```python
from build123d import *

# Parameters (mm, degrees)
CYLINDER004_R               = 7
CYLINDER004_DEPTH           = 15
CYLINDER005_R               = 7
CYLINDER005_DEPTH           = 15
BOX006_W                    = 50
BOX006_H                    = 10
BOX006_DEPTH                = 4
CYLINDER007_R               = 4.5
CYLINDER007_DEPTH           = 4
CYLINDER007_PLACEMENT_ANGLE = 15
CYLINDER006_R               = 7
CYLINDER006_DEPTH           = 4
CYLINDER006_PLACEMENT_ANGLE = 15
BOX005_W                    = 10
BOX005_H                    = 10
BOX005_DEPTH                = 10
CYLINDER002_R               = 5
CYLINDER002_DEPTH           = 45
CYLINDER002_PLACEMENT_ANGLE = 60
BOX003_W                    = 10
BOX003_H                    = 40
BOX003_DEPTH                = 5
BOX003_PLACEMENT_ANGLE      = 30
CYLINDER003_R               = 6
CYLINDER003_DEPTH           = 20
CYLINDER003_PLACEMENT_ANGLE = 25
CYLINDER_R                  = 5
CYLINDER_DEPTH              = 50
BOX001_W                    = 50
BOX001_H                    = 40
BOX001_DEPTH                = 17
BOX001_PLACEMENT_ANGLE      = 30
BOX_W                       = 50
BOX_H                       = 40
BOX_DEPTH                   = 20
BOX004_W                    = 10
BOX004_H                    = 10
BOX004_DEPTH                = 10
CYLINDER001_R               = 5
CYLINDER001_DEPTH           = 45
CYLINDER001_PLACEMENT_ANGLE = 60
BOX002_W                    = 10
BOX002_H                    = 40
BOX002_DEPTH                = 5
BOX002_PLACEMENT_ANGLE      = 30


with BuildPart() as cylinder004:
    # Cylinder004 → Cylinder004 (new body)
    with BuildSketch(Plane(origin=(0, 36, 17), x_dir=(0, 0, -1), z_dir=(1, 0, 0))):
        Circle(CYLINDER004_R)
    extrude(amount=CYLINDER004_DEPTH)


with BuildPart() as cylinder005:
    # Cylinder005 → Cylinder005 (new body)
    with BuildSketch(Plane(origin=(35, 36, 17), x_dir=(0, 0, -1), z_dir=(1, 0, 0))):
        Circle(CYLINDER005_R)
    extrude(amount=CYLINDER005_DEPTH)


with BuildPart() as cube006:
    # Box006 → Box006 (new body)
    with BuildSketch(Plane(origin=(0, 40, 0), x_dir=(1, 0, 0), z_dir=(0, 0, 1))):
        with Locations((25, 5)):
            Rectangle(BOX006_W, BOX006_H)
    extrude(amount=BOX006_DEPTH)


with BuildPart() as cylinder007:
    # Cylinder007 → Cylinder007 (new body)
    with BuildSketch(Plane.XY):
        Circle(CYLINDER007_R)
    extrude(amount=CYLINDER007_DEPTH)


with BuildPart() as cylinder007_1:
    # Cylinder007 placement: moved
    add(cylinder007.part.moved(Location((25, 43.7, 16.5))).rotate(Axis((25, 43.7, 16.5), (1, 0, 0)), CYLINDER007_PLACEMENT_ANGLE))


with BuildPart() as cut006:
    # Cylinder006 → Cylinder006 (new body)
    with BuildSketch(Plane.XY):
        Circle(CYLINDER006_R)
    extrude(amount=CYLINDER006_DEPTH)


with BuildPart() as cut006_1:
    # Cylinder006 placement: moved
    add(cut006.part.moved(Location((25, 43.7, 16.5))).rotate(Axis((25, 43.7, 16.5), (1, 0, 0)), CYLINDER006_PLACEMENT_ANGLE))

    # Cut006: cut Cylinder007
    add(cylinder007_1.part, mode=Mode.SUBTRACT)


with BuildPart() as cube005:
    # Box005 → Box005 (new body)
    with BuildSketch(Plane(origin=(40, 27, 22), x_dir=(1, 0, 0), z_dir=(0, 0, 1))):
        with Locations((5, 5)):
            Rectangle(BOX005_W, BOX005_H)
    extrude(amount=BOX005_DEPTH)


with BuildPart() as cylinder002:
    # Cylinder002 → Cylinder002 (new body)
    with BuildSketch(Plane.XY):
        Circle(CYLINDER002_R)
    extrude(amount=CYLINDER002_DEPTH)


with BuildPart() as cylinder002_1:
    # Cylinder002 placement: moved
    add(cylinder002.part.moved(Location((39, -5, 4))).rotate(Axis((39, -5, 4), (-1, 0, 0)), CYLINDER002_PLACEMENT_ANGLE))


with BuildPart() as cut004:
    # Box003 → Box003 (new body)
    with BuildSketch(Plane.XY):
        with Locations((5, 20)):
            Rectangle(BOX003_W, BOX003_H)
    extrude(amount=BOX003_DEPTH)


with BuildPart() as cut004_1:
    # Box003 placement: moved
    add(cut004.part.moved(Location((40, 0, 0))).rotate(Axis((40, 0, 0), (1, 0, 0)), BOX003_PLACEMENT_ANGLE))

    # Cut002: cut Cylinder002
    add(cylinder002_1.part, mode=Mode.SUBTRACT)

    # Cut004: cut Cube005
    add(cube005.part, mode=Mode.SUBTRACT)


with BuildPart() as cylinder003:
    # Cylinder003 → Cylinder003 (new body)
    with BuildSketch(Plane.XY):
        Circle(CYLINDER003_R)
    extrude(amount=CYLINDER003_DEPTH)


with BuildPart() as cylinder003_1:
    # Cylinder003 placement: moved
    add(cylinder003.part.moved(Location((25, 48, 12))).rotate(Axis((25, 48, 12), (1, 0, 0)), CYLINDER003_PLACEMENT_ANGLE))


with BuildPart() as cylinder:
    # Cylinder → Cylinder (new body)
    with BuildSketch(Plane(origin=(0, 36, 17), x_dir=(0, 0, -1), z_dir=(1, 0, 0))):
        Circle(CYLINDER_R)
    extrude(amount=CYLINDER_DEPTH)


with BuildPart() as cube001:
    # Box001 → Box001 (new body)
    with BuildSketch(Plane.XY):
        with Locations((25, 20)):
            Rectangle(BOX001_W, BOX001_H)
    extrude(amount=BOX001_DEPTH)


with BuildPart() as cube001_1:
    # Box001 placement: moved
    add(cube001.part.moved(Location((0, 0, 1.5))).rotate(Axis((0, 0, 1.5), (1, 0, 0)), BOX001_PLACEMENT_ANGLE))


with BuildPart() as cut005:
    # Box → Box (new body)
    with BuildSketch(Plane.XY):
        with Locations((25, 20)):
            Rectangle(BOX_W, BOX_H)
    extrude(amount=BOX_DEPTH)

    # Cut: cut Cube001
    add(cube001_1.part, mode=Mode.SUBTRACT)

    # Fusion: union Cylinder
    add(cylinder.part)

    # Cut005: cut Cylinder003
    add(cylinder003_1.part, mode=Mode.SUBTRACT)


with BuildPart() as cube004:
    # Box004 → Box004 (new body)
    with BuildSketch(Plane(origin=(0, 27, 22), x_dir=(1, 0, 0), z_dir=(0, 0, 1))):
        with Locations((5, 5)):
            Rectangle(BOX004_W, BOX004_H)
    extrude(amount=BOX004_DEPTH)


with BuildPart() as cylinder001:
    # Cylinder001 → Cylinder001 (new body)
    with BuildSketch(Plane.XY):
        Circle(CYLINDER001_R)
    extrude(amount=CYLINDER001_DEPTH)


with BuildPart() as cylinder001_1:
    # Cylinder001 placement: moved
    add(cylinder001.part.moved(Location((11, -5, 4))).rotate(Axis((11, -5, 4), (-1, 0, 0)), CYLINDER001_PLACEMENT_ANGLE))


with BuildPart() as fusion002:
    # Box002 → Box002 (new body)
    with BuildSketch(Plane.XY):
        with Locations((5, 20)):
            Rectangle(BOX002_W, BOX002_H)
    extrude(amount=BOX002_DEPTH)


with BuildPart() as fusion002_1:
    # Box002 placement: moved
    add(fusion002.part.rotate(Axis((0, 0, 0), (1, 0, 0)), BOX002_PLACEMENT_ANGLE))

    # Cut001: cut Cylinder001
    add(cylinder001_1.part, mode=Mode.SUBTRACT)

    # Cut003: cut Cube004
    add(cube004.part, mode=Mode.SUBTRACT)

    # Fusion001: union Cut004, Cut005
    add(cut004_1.part)
    add(cut005.part)

    # Fusion002: union Cylinder004, Cylinder005, Cube006, Cut006
    add(cylinder004.part)
    add(cylinder005.part)
    add(cube006.part)
    add(cut006_1.part)


solid = fusion002_1.part
```
The model under review builds one solid part; all positions refer to its coordinate system, in mm. A direction names the side the tool comes from. Give positions to 0.01 mm unless a question says otherwise; leave off trailing zeros. Write each loop counter-clockwise with the first axis right and the second up, starting at its lowest first coordinate (ties: lowest second). Pieces come first, ordered by that corner, then holes. Notation, with made-up numbers: M 87.25,-33.5 L 136.25,-33.5 A30 ccw 136.25,-11.5 Z; hole C 20,-33.75 d8. An arc over 180 degrees is marked long. Write item = value, one per line. Start each with the question number.
Q1. Clearance check with flat-ended pins moving along their axes: pin 1 (11 mm diameter, centred on x = 29, y = 47.5, fed in from +Z); pin 2 (3 mm diameter, centred on y = 41.5, z = 18.5, fed in from -X); pin 3 (2 mm diameter, centred on x = 24, y = 9, fed in from +Z); pin 4 (3 mm diameter, centred on x = 37, z = 2, fed in from +Y). State where each tip first meets the part, or that it passes through.
Q2. We need section A-A (x = 27). State the section outline as (y, z) points.
Q3. We need section B-B (x = 4). State the section outline as (y, z) points.
Q4. Machinability: for faces 1 (the face through (3.82, -1.23, 2.13)), 2 (the face through (43.002, 14.713, 11.92)), 3 (the face through (24.9, 47.61, 21.69)), 4 (the face through (24.902, 48.909, 17.896)), 5 (the face through (3, 30, 22)), which of the approach directions +Z, -Z, +X, -X, +Y, -Y give a long, thin tool a straight path to every point of the face, cutting with its end or side? Answer none if there is none.
Q5. We need section C-C (y = 36). State the section outline as (x, z) points, plus the area to 3 significant figures.
Q6. Mouldability with a two-part tool opening along Z and no side actions: class faces 6 (the face through (46.04, -1.23, 2.13)), 7 (the face through (42.395, 39.971, 22.765)), 8 (the face through (50, 23, 9)) as released by +Z, released by -Z, zero draft, split by the parting line, or undercut.
Q7. For line 1 (Y direction, x = 14, z = 1.5); line 2 (X direction, y = 14, z = 12.75); line 3 (X direction, y = 10, z = 8.5), list the stretches that pass through material, from the lowest coordinate up.
Result set:
q1.pin_1 = 22.18
q1.pin_2 = 0
q1.pin_3 = 7.27
q1.pin_4 = 50
q2.outline = M 0,0 L 50,0 L 50,4 L 40,4 L 40,14 A5 ccw 40.47,14.76 L 39.35,17.17 L 38.77,19.32 L 38.39,19.22 L 37.16,21.86 A5 ccw 31.97,19.96 L 0,1.5 Z; M 46.56,21.41 L 47.59,17.54 L 50.18,18.24 L 49.14,22.1 Z
q3.outline = M -2.5,4.33 L 0,0 L 50,0 L 50,4 L 40,4 L 40,11.26 A7 ccw long 31.1,22 L 28.11,22 Z
q4.face_1 = -Z, +X, -X, -Y
q4.face_2 = +Z, -Y
q4.face_3 = +Z
q4.face_4 = +Y
q4.face_5 = +Z, +X, -X, -Y
q5.outline = M 0,0 L 50,0 L 50,24 L 35,24 L 35,22 L 15,22 L 15,24 L 0,24 Z
q5.area = 1,160 mm2
q6.face_6 = released by -Z
q6.face_7 = undercut
q6.face_8 = zero draft
q7.line_1 = 0 to 50
q7.line_2 = 0 to 6.38, 43.62 to 50
q7.line_3 = 0 to 7.53, 42.47 to 50
